```python
from build123d import *

# Parameters (mm, degrees)
F0_W     = 90
F0_H     = 45
F1_DEPTH = 41
F2_R     = 17.5
F3_DEPTH = 80.040589
F5_DEPTH = 60
F6_R     = 17.5
F7_DEPTH = 28.8


with BuildPart() as f1:
    # F0 (on Front) → F1 (new body)
    with BuildSketch(Plane.XZ):
        Rectangle(F0_W, F0_H)
    extrude(amount=F1_DEPTH)

    # F2 (on Front) → F3 (cut)
    with BuildSketch(Plane.XZ):
        with Locations((-7.5, 0)):
            Circle(F2_R)
    extrude(amount=F3_DEPTH, mode=Mode.SUBTRACT)

    # F4 (on face) → F5 (cut, symmetric)
    with BuildSketch(Plane.XZ):
        Polygon((-20.405538, 34.710526), (50.253086, -8.42718), (50.312012, 38.423195), align=None)
    extrude(amount=F5_DEPTH, both=True, mode=Mode.SUBTRACT)

    # F6 (on face) → F7 (cut)
    with BuildSketch(Plane(origin=(-45, 0, 0), x_dir=(0, -1, 0), z_dir=(-1, 0, 0))):
        with Locations((20.5, 0)):
            Circle(F6_R)
    extrude(amount=-F7_DEPTH, mode=Mode.SUBTRACT)


solid = f1.part
```
Geometry check sheet. Reference: the model listing, model coordinates, mm. A direction names the side the tool comes from. Round coordinates to 2 decimals unless told otherwise and drop trailing zeros. Order: outer loops, then holes, each group sorted by start corner. A loop starts at its lowest first (then second) coordinate and runs counter-clockwise, first axis right, second up. Notation, with made-up numbers: (72.5, 0) - (92.5, 0) arc R14 cw to (92.5, 11) - close; hole circle Ø3 at (-32.5, 60). An arc over 180 degrees is marked (long way). Use a Markdown table: item, result. Add a question column.
1) Gauge pin test, flat ends, axial feed: P1, Ø10, axis at y = -27.5, z = -4, coming from the -X side; P2, Ø4, axis at y = -6, z = -5, coming from the -X side. Record the tip position at first contact, or that the pin passes through.
2) Set-up check for faces 4 (the flat face through (-16.2, -20, -16)), 5 (the flat face through (9, -41, -10)): record each of +Z, -Z, +X, -X, +Y, -Y from which the full face is reachable in a straight line by a thin tool's end or side.
3) Section check C-C (y = -20.5). Record the cut outline in (x, z), then the cut area to 3 significant figures.
4) Thickness scan on line 1 along Z through (x, y) = (-7.5, -8.5); line 2 along Y through (x, z) = (-31, 0); line 3 along X through (y, z) = (-26, 15.5). Record the ranges inside material, lowest first.
5) Section check B-B (x = -7.5). Record the cut outline in (y, z).
6) Section check D-D (z = -2.5). Record the cut outline in (x, y), then the cut area to 3 significant figures.
7) Mould release check, pull along X, two halves, no side actions. Record for faces 1 (the flat face through (-16.2, -20, 16)), 2 (the flat face through (21.98, -20.787, 8.834)), 3 (the cylindrical face through (9.19, -20.21, 5.26)): released by +X, released by -X, zero draft, split by the parting line, or undercut.
8) Section check A-A (z = -10.5). Record the cut outline in (x, y), then the cut area to 3 significant figures.
Established:
| question | item | result |
|---|---|---|
| 1 | P1 | x = 7.51 |
| 1 | P2 | x = 8.54 |
| 2 | face 4 | -X |
| 2 | face 5 | +Z, -Z, +X, -X, -Y |
| 3 | outline | (-45, -22.5) - (45, -22.5) - (45, -5.22) - (-0.4, 22.5) - (-45, 22.5) - (-45, 17.5) - (-16.2, 17.5) - (-16.2, 15.18) arc R17.5 cw (long way) to (-16.2, -15.18) - (-16.2, -17.5) - (-45, -17.5) - close |
| 3 | area | 1,640 mm2 |
| 4 | line 1 | -22.5 to -17.5, 17.5 to 22.5 |
| 4 | line 2 | -41 to -38, -3 to 0 |
| 4 | line 3 | -16.2 to -15.62, 0.62 to 11.06 |
| 5 | outline | (-41, -22.5) - (0, -22.5) - (0, -17.5) - (-41, -17.5) - close; (-41, 17.5) - (0, 17.5) - (0, 22.5) - (-41, 22.5) - close |
| 6 | outline | (-45, -41) - (-24.82, -41) - (-24.82, -37.82) - (-45, -37.82) - close; (-45, -3.18) - (-24.82, -3.18) - (-24.82, 0) - (-45, 0) - close; (9.82, -41) - (40.54, -41) - (40.54, 0) - (9.82, 0) - close |
| 6 | area | 1,390 mm2 |
| 7 | face 1 | released by -X |
| 7 | face 2 | released by +X |
| 7 | face 3 | undercut |
| 8 | outline | (-45, -41) - (-21.5, -41) - (-21.5, -34.5) - (-45, -34.5) - close; (-45, -6.5) - (-21.5, -6.5) - (-21.5, 0) - (-45, 0) - close; (6.5, -41) - (45, -41) - (45, 0) - (6.5, 0) - close |
| 8 | area | 1,880 mm2 |
